The figure shows three views and two pictorial views of one solid part (mm, origin at its lowest corner). Answer the questions. Coordinates: 2 decimals unless noted, no trailing zeros. Write each loop counter-clockwise with the first axis right and the second up, starting at its lowest first coordinate (ties: lowest second). Pieces come first, ordered by that corner, then holes. Notation, with made-up numbers: (87.25, -6.75) - (131.25, -6.75) arc R33 ccw to (131.25, 24.25) - close; hole circle Ø8 at (86.5, -27.75). An arc over 180 degrees is marked (long way). Use a Markdown table: item, result. Add a question column.
(1) For a pull along X with two mould halves and no side action, classify the marked faces 1, 2 and 3 as released by +X, released by -X, zero draft, split by the parting line, or undercut.
(2) The part is cut by section A-A, the plane z = 3.25. Give the vertices of the cut face in (x, y) (3 decimals), then the cut area to 3 significant figures.
(3) The part is cut by section B-B, the plane x = 3. Give the vertices of the cut face in (y, z), then the cut area to 3 significant figures.
(4) The part is cut by section D-D, the plane x = 20. Give the vertices of the cut face in (y, z), then the cut area to 3 significant figures.
(5) The part is cut by section C-C, the plane y = 18.5. Give the vertices of the cut face in (x, z).
(6) Find the intervals of material crossed by line 1 (Y direction, x = 25, z = 2.95); line 2 (Y direction, x = 25.25, z = 0.3); line 3 (Y direction, x = 24.5, z = 3.05), in increasing order. Write a range as from..to.
(7) Given pin 1 Ø8 at (x, y) = (20.5, 15) entering from +Z, flat-ended and moving along its own axis, determine where the tip first touches the part or whether it passes through.
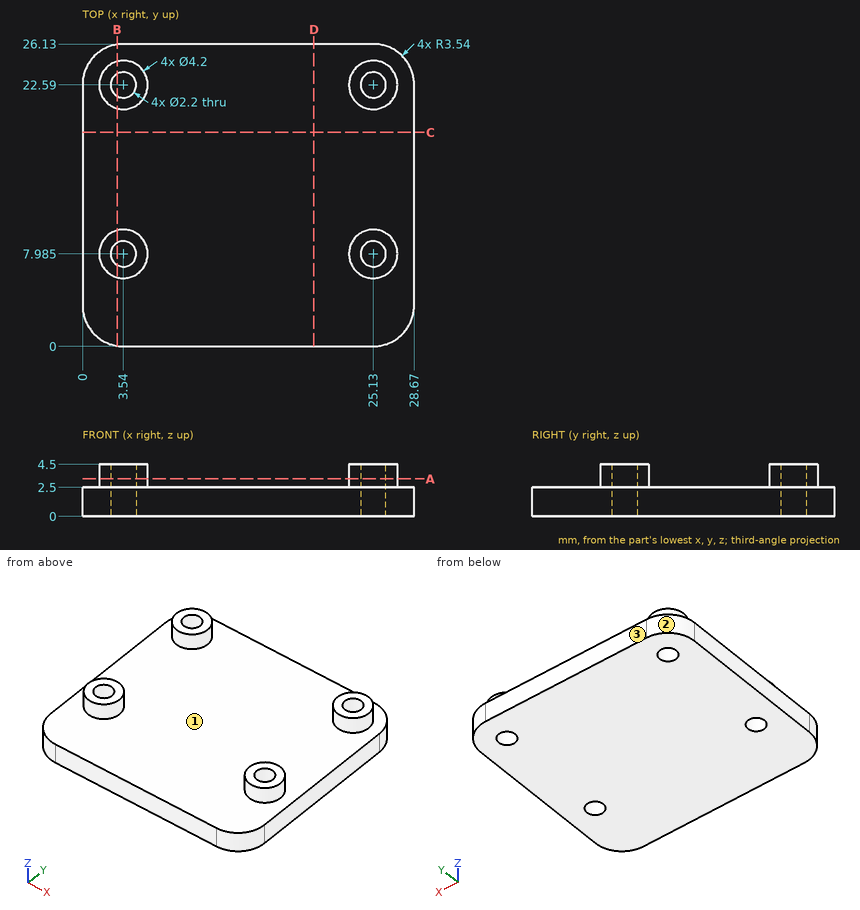
Model answer:
| question | item | result |
|---|---|---|
| 1 | face 1 | undercut |
| 1 | face 2 | released by -X |
| 1 | face 3 | zero draft |
| 2 | outline | circle Ø4.2 at (3.54, 7.985); circle Ø4.2 at (3.54, 22.59); circle Ø4.2 at (25.13, 7.985); circle Ø4.2 at (25.13, 22.59); hole circle Ø2.2 at (3.54, 7.985); hole circle Ø2.2 at (3.54, 22.59); hole circle Ø2.2 at (25.13, 7.985); hole circle Ø2.2 at (25.13, 22.59) |
| 2 | area | 40.2 mm^2 |
| 3 | outline | (0.04, 0) - (7.03, 0) - (7.03, 4.5) - (5.96, 4.5) - (5.96, 2.5) - (0.04, 2.5) - close; (8.94, 0) - (21.63, 0) - (21.63, 4.5) - (20.56, 4.5) - (20.56, 2.5) - (10.01, 2.5) - (10.01, 4.5) - (8.94, 4.5) - close; (23.55, 0) - (26.09, 0) - (26.09, 2.5) - (24.62, 2.5) - (24.62, 4.5) - (23.55, 4.5) - close |
| 3 | area | 64.1 mm^2 |
| 4 | outline | (0, 0) - (26.13, 0) - (26.13, 2.5) - (0, 2.5) - close |
| 4 | area | 65.3 mm^2 |
| 5 | outline | (0, 0) - (28.67, 0) - (28.67, 2.5) - (0, 2.5) - close |
| 6 | line 1 | 5.89..6.89, 9.08..10.08, 20.49..21.5, 23.68..24.69 |
| 6 | line 2 | 0..6.89, 9.08..21.5, 23.68..26.13 |
| 6 | line 3 | 5.98..7.08, 8.89..9.99, 20.59..21.69, 23.49..24.59 |
| 7 | pin 1 | z = 2.5 |
